CAD build for the part. Positions are in the model's coordinates, mm. A direction names the side the tool comes from. Coordinates: 2 decimals unless noted, no trailing zeros. Write each loop counter-clockwise with the first axis right and the second up, starting at its lowest first coordinate (ties: lowest second). Pieces come first, ordered by that corner, then holes.
```python
from build123d import *

# Parameters (mm, degrees)
SKETCH1_R           = 2.285
SKETCH1_R_2         = 1.5
BOSS_EXTRUDE1_DEPTH = 8


with BuildPart() as part:
    # Sketch1 → Boss-Extrude1 (new body)
    with BuildSketch(Plane(origin=(0, 0, 0), x_dir=(1, 0, 0), z_dir=(0, 1, 0))):
        Polygon((-115, 130), (115, 130), (115, 62.88), (122, 62.88), (122, -62.88), (115, -62.88), (115, -130), (-115, -130), (-115, -62.88), (-122, -62.88), (-122, 62.88), (-115, 62.88), align=None)
        with Locations(Location((-75, -112, 0), (0, 0, 270))):
            Circle(SKETCH1_R, mode=Mode.SUBTRACT)
        with Locations(Location((-97, -82, 0), (0, 0, 270))):
            Circle(SKETCH1_R, mode=Mode.SUBTRACT)
        with Locations(Location((97, -82, 0), (0, 0, 90))):
            Circle(SKETCH1_R, mode=Mode.SUBTRACT)
        with Locations(Location((75, -112, 0), (0, 0, 90))):
            Circle(SKETCH1_R, mode=Mode.SUBTRACT)
        with Locations(Location((75, 112, 0), (0, 0, 270))):
            Circle(SKETCH1_R, mode=Mode.SUBTRACT)
        with Locations(Location((97, 82, 0), (0, 0, 270))):
            Circle(SKETCH1_R, mode=Mode.SUBTRACT)
        with Locations(Location((-97, 82, 0), (0, 0, 90))):
            Circle(SKETCH1_R, mode=Mode.SUBTRACT)
        with Locations(Location((-75, 112, 0), (0, 0, 90))):
            Circle(SKETCH1_R, mode=Mode.SUBTRACT)
        with Locations(Location((-114.5, 50.875, 0), (0, 0, 270))):
            Circle(SKETCH1_R_2, mode=Mode.SUBTRACT)
        with Locations(Location((-97.5, 50.875, 0), (0, 0, 270))):
            Circle(SKETCH1_R_2, mode=Mode.SUBTRACT)
        with Locations(Location((-114.5, -50.875, 0), (0, 0, 270))):
            Circle(SKETCH1_R_2, mode=Mode.SUBTRACT)
        with Locations(Location((-97.5, -50.875, 0), (0, 0, 270))):
            Circle(SKETCH1_R_2, mode=Mode.SUBTRACT)
        with Locations(Location((97.5, -50.875, 0), (0, 0, 90))):
            Circle(SKETCH1_R_2, mode=Mode.SUBTRACT)
        with Locations(Location((114.5, -50.875, 0), (0, 0, 90))):
            Circle(SKETCH1_R_2, mode=Mode.SUBTRACT)
        with Locations(Location((97.5, 50.875, 0), (0, 0, 90))):
            Circle(SKETCH1_R_2, mode=Mode.SUBTRACT)
        with Locations(Location((114.5, 50.875, 0), (0, 0, 90))):
            Circle(SKETCH1_R_2, mode=Mode.SUBTRACT)
        with BuildLine():
            Line((-76.605976208, 4.735064986), (73.394023792, 55.610064986))
            ThreePointArc((73.394023792, 55.610064986), (79.735064986, 52.480976208), (76.605976208, 46.139935014))
            Line((76.605976208, 46.139935014), (-73.394023792, -4.735064986))
            ThreePointArc((-73.394023792, -4.735064986), (-79.735064986, -1.605976208), (-76.605976208, 4.735064986))
        make_face(mode=Mode.SUBTRACT)
        with BuildLine():
            Line((-76.605976208, -46.139935014), (73.394023792, 4.735064986))
            ThreePointArc((73.394023792, 4.735064986), (79.735064986, 1.605976208), (76.605976208, -4.735064986))
            Line((76.605976208, -4.735064986), (-73.394023792, -55.610064986))
            ThreePointArc((-73.394023792, -55.610064986), (-79.735064986, -52.480976208), (-76.605976208, -46.139935014))
        make_face(mode=Mode.SUBTRACT)
    extrude(amount=BOSS_EXTRUDE1_DEPTH)


solid = part.part
```
Item 1: Saw through at B-B, the plane z = 39.5. Write the cut outline in (x, y).
Item 2: Which spindle directions (+Z, -Z, +X, -X, +Y, -Y) get a long thin tool onto all of the face, cutting with end or side? Do faces 4 (the flat face through (-118, 4, 62.88)), 5 (the flat face through (119, 4, 62.88)), 6 (the flat face through (118, 4, -62.88)), 7 (the flat face through (2.66, 3.94, -21.06)). Say none if no direction does.
Item 3: Flat gauge pins, fed straight in: pin 1 Ø2 at (x, y) = (-117.5, 4) entering from +Z; pin 2 Ø1.8 at (x, z) = (-114.5, 50.875) entering from +Y; pin 3 Ø3.5 at (x, y) = (-117.5, 4) entering from -Z; pin 4 Ø1.5 at (y, z) = (7, 93.5) entering from -X. Where does each tip first touch, or does it go through?
Item 4: Saw through at A-A, the plane z = 0. Write the cut outline in (x, y).
Item 5: Two-plate mould, pull along X, no slides. Class faces 1 (the flat face through (2.7, 3.9, 29.8)), 2 (the flat face through (2, 0, -2)), 3 (the flat face through (-115, 4, 97)): +X half, -X half, draft (parallel to the pull), parting line (faces both ways), or undercut.
Item 6: Wall check: line 1 along Z through (x, y) = (114.5, 5) (3 decimals); line 2 along X through (y, z) = (1.75, 111.5); line 3 along X through (y, z) = (2.25, 82) (3 decimals). Give the ranges that are in metal, low to high.
Item 7: Saw through at C-C, the plane y = 5.5. State how many separate pieces and enclosed holes the cut face has, and give its area (3 significant figures).
Item 8: Saw through at D-D, the plane z = -66. Write the cut outline in (x, y), and give its area (3 significant figures).
Working result:
1. outline: (-122, 0) - (-57.03, 0) - (-57.03, 8) - (-122, 8) - close; (-25.9, 0) - (122, 0) - (122, 8) - (-25.9, 8) - close
2. face 4: +Z, -X, +Y, -Y
2. face 5: +Z, +X, +Y, -Y
2. face 6: -Z, +X, +Y, -Y
2. face 7: +Y, -Y
3. pin 1: stops at z = 62.88
3. pin 2: passes through
3. pin 3: stops at z = -62.88
3. pin 4: stops at x = -115
4. outline: (-122, 0) - (-80, 0) - (-80, 8) - (-122, 8) - close; (-59.43, 0) - (59.43, 0) - (59.43, 8) - (-59.43, 8) - close; (80, 0) - (122, 0) - (122, 8) - (80, 8) - close
5. face 1: undercut
5. face 2: draft
5. face 3: -X half
6. line 1: z = -130 to -52.375, -49.375 to 49.375, 52.375 to 130
6. line 2: x = -115 to -77.23, -72.77 to 72.77, 77.23 to 115
6. line 3: x = -115 to -99.285, -94.715 to 94.715, 99.285 to 115
7. separate pieces: 1
7. enclosed holes: 18
7. area: 58,000 mm2
8. outline: (-115, 0) - (115, 0) - (115, 8) - (-115, 8) - close
8. area: 1,840 mm2
